Input: dimensioned drawing with shaded views. Units: mm. Origin: part minimum x, y, z. Give positions to 0.01 mm unless a question says otherwise; leave off trailing zeros. Loops run counter-clockwise (first coordinate to the right, second up) from the corner with the lowest first, then second, coordinate; pieces in that order, holes last.
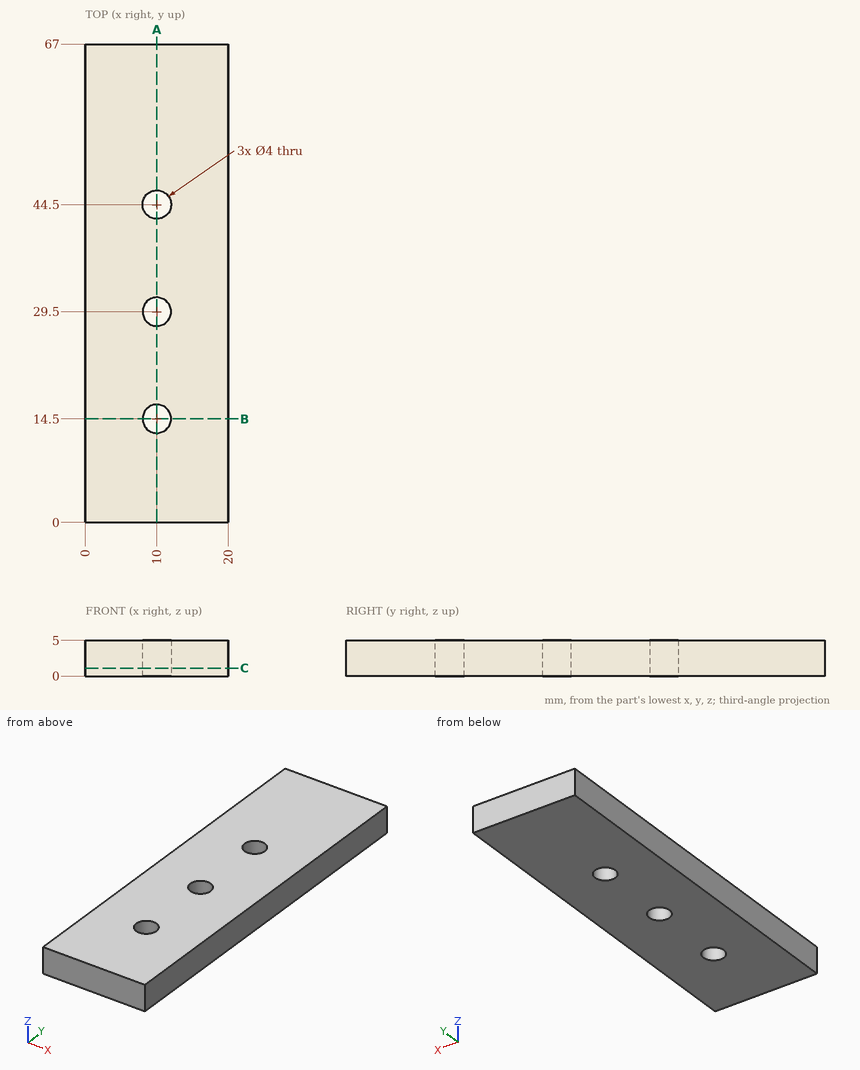
(1) Section A-A, the plane x = 10. Return the cut outline in (y, z), then the cut area to 3 significant figures.
A:
outline: (0, 0) - (12.5, 0) - (12.5, 5) - (0, 5) - close; (16.5, 0) - (27.5, 0) - (27.5, 5) - (16.5, 5) - close; (31.5, 0) - (42.5, 0) - (42.5, 5) - (31.5, 5) - close; (46.5, 0) - (67, 0) - (67, 5) - (46.5, 5) - close
area: 275 mm2
(2) Section C-C, the plane z = 1.1. Return the cut outline in (x, y).
A:
outline: (0, 0) - (20, 0) - (20, 67) - (0, 67) - close; hole circle Ø4 at (10, 14.5); hole circle Ø4 at (10, 29.5); hole circle Ø4 at (10, 44.5)
(3) Section B-B, the plane y = 14.5. Return the cut outline in (x, z), then the cut area to 3 significant figures.
A:
outline: (0, 0) - (8, 0) - (8, 5) - (0, 5) - close; (12, 0) - (20, 0) - (20, 5) - (12, 5) - close
area: 80.0 mm2
(4) Ray query, line 1 along Y through (x, z) = (10, 1.3); line 2 along Y through (x, z) = (8.5, 2.35); line 3 along X through (y, z) = (28.5, 0.55). Return the intervals inside material, ascending.
A:
line 1: y = 0 to 12.5, 16.5 to 27.5, 31.5 to 42.5, 46.5 to 67
line 2: y = 0 to 13.18, 15.82 to 28.18, 30.82 to 43.18, 45.82 to 67
line 3: x = 0 to 8.27, 11.73 to 20
